from build123d import *
from build123d.topology import SkipClean

# Parameters (mm, degrees)
SKETCH1_R           = 12.25
BOSS_EXTRUDE1_DEPTH = 1.05
BOSS_EXTRUDE2_START = 2.1
BOSS_EXTRUDE2_DEPTH = 2.1
BOSS_EXTRUDE3_DEPTH = 2.1


with BuildPart() as part:
    # Sketch1 → Boss-Extrude1 (new, symmetric)
    with BuildSketch(Plane.XY):
        Circle(SKETCH1_R)
    extrude(amount=BOSS_EXTRUDE1_DEPTH, both=True)

    # Sketch2 → Boss-Extrude2 (add)
    with SkipClean():  # the faces are left unmerged after this step: merging them gives an invalid solid
        with BuildSketch(Plane.XY.offset(1.05).offset(BOSS_EXTRUDE2_START)):
            with BuildLine():
                Line((-12.124355653, 1.75), (12.124355653, 1.75))
                ThreePointArc((12.124355653, 1.75), (12.25, 0), (12.124355653, -1.75))
                Line((12.124355653, -1.75), (-12.124355653, -1.75))
                ThreePointArc((-12.124355653, -1.75), (-12.25, 0), (-12.124355653, 1.75))
            make_face()
        extrude(amount=-BOSS_EXTRUDE2_DEPTH)

    # Sketch3 → Boss-Extrude3 (add)
    with SkipClean():  # the faces are left unmerged after this step: merging them gives an invalid solid
        with BuildSketch(Plane(origin=(0, 0, -1.05), x_dir=(-1, 0, 0), z_dir=(0, 0, -1))):
            with BuildLine():
                Line((-1.75, -12.124355653), (-1.75, 12.124355653))
                ThreePointArc((-1.75, 12.124355653), (0, 12.25), (1.75, 12.124355653))
                Line((1.75, 12.124355653), (1.75, -12.124355653))
                ThreePointArc((1.75, -12.124355653), (0, -12.25), (-1.75, -12.124355653))
            make_face()
        extrude(amount=BOSS_EXTRUDE3_DEPTH)


solid = part.part
Read the model definition and answer for the solid it produces. Units are mm, in the model's axes. A direction names the side the tool comes from. Round coordinates to 2 decimals unless told otherwise and drop trailing zeros. Write each loop counter-clockwise with the first axis right and the second up, starting at its lowest first coordinate (ties: lowest second). Pieces come first, ordered by that corner, then holes.
1. The part is cut by section C-C, the plane z = 1.5. Determine the outline of the cut face in (x, y).
2. The part is cut by section B-B, the plane x = 0. Determine the outline of the cut face in (y, z).
3. The part is cut by section A-A, the plane y = 0. Determine the outline of the cut face in (x, z).
4. Straight lines are drawn through the part: L1, parallel to Z at x = -10.5, y = -3.5; L2, parallel to X at y = -2.5, z = -1.75. For each, find the intervals that lie inside material, in ascending order.
5. The part is cut by section D-D, the plane z = -0.5. Determine the outline of the cut face in (x, y), then the cut area to 3 significant figures.
6. Which of the six approach directions +Z, -Z, +X, -X, +Y, -Y give full straight-line access (tool end or side, diameter ignored) to faces 1 (the face through (-6, 0, -1.05)), 2 (the face through (0, -6, 1.05)), 3 (the face through (1.75, 0, -2))?
7. Given pin 1 Ø1.7 at (x, z) = (-5, 2.5) entering from -Y; pin 2 Ø2.5 at (x, z) = (1.5, 2) entering from +Y; pin 3 Ø1.1 at (y, z) = (-2, -2.5) entering from -X, each flat-ended and moving along its own axis, determine where each tip first touches the part or whether it passes through.
Values:
1. outline: (-12.12, -1.75) - (12.12, -1.75) arc R12.25 ccw to (12.12, 1.75) - (-12.12, 1.75) arc R12.25 ccw to start
2. outline: (-12.25, -3.15) - (12.25, -3.15) - (12.25, 1.05) - (1.75, 1.05) - (1.75, 3.15) - (-1.75, 3.15) - (-1.75, 1.05) - (-12.25, 1.05) - close
3. outline: (-12.25, -1.05) - (-1.75, -1.05) - (-1.75, -3.15) - (1.75, -3.15) - (1.75, -1.05) - (12.25, -1.05) - (12.25, 3.15) - (-12.25, 3.15) - close
4. L1: z = -1.05 to 1.05
4. L2: x = -1.75 to 1.75
5. outline: circle Ø24.5 at (0, 0)
5. area: 471 mm2
6. face 1: -Z, -X, +Y, -Y
6. face 2: +Z, +X, -X, -Y
6. face 3: -Z, +X, +Y, -Y
7. pin 1: stops at y = -1.75
7. pin 2: stops at y = 12.23
7. pin 3: stops at x = -1.75
